```python
from build123d import *

# Parameters (mm, degrees)
SKETCH4_W           = 5
SKETCH4_H           = 70
BOSS_EXTRUDE1_DEPTH = 64.5
FILLET3_R           = 10
FILLET4_R           = 10
SKETCH5_R           = 21.9509271
CUT_EXTRUDE1_DEPTH  = 10


with BuildPart() as part:
    # Sketch4 → Boss-Extrude1 (new body)
    with BuildSketch(Plane.XY):
        with Locations((-0.263157895, -27.861842105)):
            Rectangle(SKETCH4_W, SKETCH4_H)
    extrude(amount=BOSS_EXTRUDE1_DEPTH)

    # Fillet3
    fillet3_edges = [part.edges().sort_by_distance(p)[0] for p in [
        (-0.263157895, 7.138157895, 64.5),
    ]]
    fillet(fillet3_edges, radius=FILLET3_R)

    # Fillet4
    fillet4_edges = [part.edges().sort_by_distance(p)[0] for p in [
        (-0.263157895, 7.138157895, 0),
    ]]
    fillet(fillet4_edges, radius=FILLET4_R)

    # Sketch5 → Cut-Extrude1 (cut)
    with BuildSketch(Plane.ZY.offset(2.763157895)):
        with Locations((31.75, -27.861842105)):
            Circle(SKETCH5_R)
    extrude(amount=-CUT_EXTRUDE1_DEPTH, mode=Mode.SUBTRACT)


solid = part.part
```
The listing builds one solid part. Answer for the finished solid, in the listing's coordinates (mm). Coordinates: 2 decimals unless noted, no trailing zeros. Write each loop counter-clockwise with the first axis right and the second up, starting at its lowest first coordinate (ties: lowest second). Pieces come first, ordered by that corner, then holes.
Q1. Section A-A, the plane z = 31.75 is taken. Write down the section's boundary in (x, y), then the cut area to 3 significant figures.
Returned:
outline: (-2.76, -62.86) - (2.24, -62.86) - (2.24, -49.81) - (-2.76, -49.81) - close; (-2.76, -5.91) - (2.24, -5.91) - (2.24, 7.14) - (-2.76, 7.14) - close
area: 130 mm2
Q2. The mould has two halves that part along Y. Classify faces 1 (the cylindrical face through (-0.23, 4.29, 61.49)), 2 (the flat face through (0, -32, 64.5)), 3 (the cylindrical face through (-0.3, -49.29, 26.99)): released by +Y, released by -Y, zero draft, split by the parting line, or undercut.
Returned:
face 1: released by +Y
face 2: zero draft
face 3: undercut
Q3. Find the intervals of material crossed by line 1 along Y through (x, z) = (0.65, 31.75); line 2 along Z through (x, y) = (-0.35, -28.5); line 3 along Y through (x, z) = (-1.6, 37), in increasing order.
Returned:
line 1: y = -62.86 to -49.81, -5.91 to 7.14
line 2: z = 0 to 9.81, 53.69 to 64.5
line 3: y = -62.86 to -49.18, -6.55 to 7.14
Q4. Section B-B, the plane y = -9 is taken. Write down the section's boundary in (x, z), then the cut area to 3 significant figures.
Returned:
outline: (-2.76, 0) - (2.24, 0) - (2.24, 20.52) - (-2.76, 20.52) - close; (-2.76, 42.98) - (2.24, 42.98) - (2.24, 64.5) - (-2.76, 64.5) - close
area: 210 mm2
Q5. Section C-C, the plane x = -1.55 is taken. Write down the section's boundary in (y, z).
Returned:
outline: (-62.86, 0) - (-2.86, 0) arc R10 ccw to (7.14, 10) - (7.14, 54.5) arc R10 ccw to (-2.86, 64.5) - (-62.86, 64.5) - close; hole circle Ø43.9 at (-27.86, 31.75)
